from build123d import *

# Parameters (mm, degrees)
SKETCH_1_W               = 114
SKETCH_1_H               = 15
EXTRUDE_1_DEPTH          = 114
FILLET_3_R               = 15
FILLET_4_R               = 2
SKETCH_2_R               = 24
EXTRUDE_2_DEPTH          = 43
FILLET_5_R               = 12
SKETCH_3_R               = 6.5
CUT_EXTRUDE_4_DEPTH      = 167.856225604
SKETCH_3_4_R             = 11
SKETCH_3_4_R_2           = 6.5
CUT_EXTRUDE_5_DEPTH      = 1.5
PATTERN_CIRCULAR_1_COUNT = 4


with BuildPart() as part:
    # Sketch 1 → Extrude 1 (new body)
    with BuildSketch(Plane.XY):
        with Locations((57, -7.5)):
            Rectangle(SKETCH_1_W, SKETCH_1_H)
    extrude(amount=-EXTRUDE_1_DEPTH)

    # Fillet 3
    fillet_3_edges = [part.edges().sort_by_distance(p)[0] for p in [
        (114, -7.5, -114),
        (0, -7.5, -114),
        (114, -7.5, 0),
        (0, -7.5, 0),
    ]]
    fillet(fillet_3_edges, radius=FILLET_3_R)

    # Fillet 4
    fillet_4_edges = [part.edges().sort_by_distance(p)[0] for p in [
        (0, 0, -57),
        (57, 0, -114),
        (57, 0, 0),
        (114, 0, -57),
        (109.606601718, 0, -4.393398282),
        (109.606601718, 0, -109.606601718),
        (4.393398282, 0, -4.393398282),
        (4.393398282, 0, -109.606601718),
    ]]
    fillet(fillet_4_edges, radius=FILLET_4_R)

    # Sketch 2 → Extrude 2 (add)
    with BuildSketch(Plane(origin=(0, 0, 0), x_dir=(1, 0, 0), z_dir=(0, 1, 0))):
        with Locations(Location((57, 57, 0), (0, 0, 270))):
            Circle(SKETCH_2_R)
        with BuildLine():
            ThreePointArc((47.050125629, 56), (67, 57), (47.050125629, 58))
            Line((47.050125629, 58), (43.8, 58))
            Line((43.8, 58), (43.8, 56))
            Line((43.8, 56), (47.050125629, 56))
        make_face(mode=Mode.SUBTRACT)
    extrude(amount=EXTRUDE_2_DEPTH)

    # Fillet 5
    fillet_5_edges = [part.edges().sort_by_distance(p)[0] for p in [
        (57, 0, -81),
    ]]
    fillet(fillet_5_edges, radius=FILLET_5_R)

    # Sketch 3 → Cut-Extrude 4 (cut, through all)
    with BuildSketch(Plane(origin=(0, 0, 0), x_dir=(1, 0, 0), z_dir=(0, 1, 0))):
        with Locations(Location((99, 99.206255551, 0), (0, 0, 270))):
            Circle(SKETCH_3_R)
    cut_extrude_4 = extrude(amount=-CUT_EXTRUDE_4_DEPTH, mode=Mode.SUBTRACT)

    # Sketch 3_4 → Cut-Extrude 5 (cut)
    with BuildSketch(Plane(origin=(0, 0, 0), x_dir=(1, 0, 0), z_dir=(0, 1, 0))):
        with Locations(Location((99, 99.206255551, 0), (0, 0, 270))):
            Circle(SKETCH_3_4_R)
        with Locations(Location((99, 99.206255551, 0), (0, 0, 270))):
            Circle(SKETCH_3_4_R_2, mode=Mode.SUBTRACT)
    cut_extrude_5 = extrude(amount=-CUT_EXTRUDE_5_DEPTH, mode=Mode.SUBTRACT)

    # Pattern Circular 1: Cut-Extrude 4, Cut-Extrude 5 ×4 about axis
    pattern_circular_1_axis = Axis((57, 0, -57), (0, 1, 0))
    add([cut_extrude_4.rotate(pattern_circular_1_axis, i * 360 / PATTERN_CIRCULAR_1_COUNT) for i in range(1, PATTERN_CIRCULAR_1_COUNT)], mode=Mode.SUBTRACT)
    add([cut_extrude_5.rotate(pattern_circular_1_axis, i * 360 / PATTERN_CIRCULAR_1_COUNT) for i in range(1, PATTERN_CIRCULAR_1_COUNT)], mode=Mode.SUBTRACT)


solid = part.part
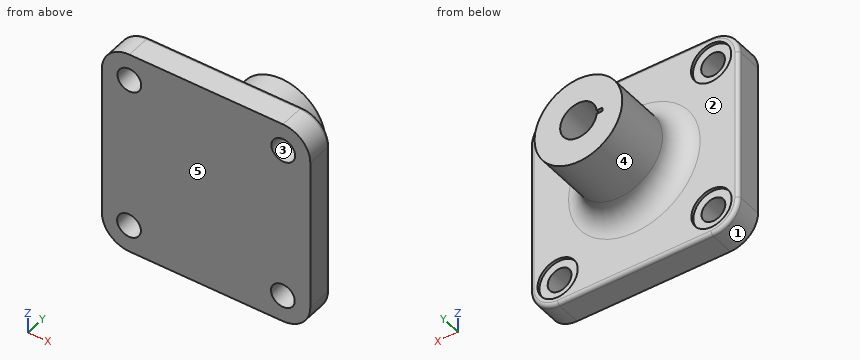
Work out the finished part from the listing and answer in its coordinate system (mm). Face numbers are marked on the shaded views. A direction names the side the tool comes from. Give positions to 0.01 mm unless a question says otherwise; leave off trailing zeros. Loops run counter-clockwise (first coordinate to the right, second up) from the corner with the lowest first, then second, coordinate; pieces in that order, holes last. Notation, with made-up numbers: (-5.5, 45) - (48.5, 45) arc R20 ccw to (48.5, 67) - close; hole circle Ø1 at (72.5, -35). An arc over 180 degrees is marked (long way). Answer in a Markdown table with one row per item.
(1) Section B-B (y = 19.5) is taken. Give the vertices of the cut face in (x, z).
Results list:
| item | result |
|---|---|
| outline | circle Ø48 at (57, -57); hole (43.8, -58) - (47.05, -58) arc R10 ccw (long way) to (47.05, -56) - (43.8, -56) - close |
(2) Section D-D (x = 57) is taken. Give the vertices of the cut face in (y, z).
Results list:
| item | result |
|---|---|
| outline | (-15, -114) - (-2, -114) arc R2 ccw to (0, -112) - (0, -93) arc R12 cw to (12, -81) - (43, -81) - (43, -67) - (0, -67) - (0, -47) - (43, -47) - (43, -33) - (12, -33) arc R12 cw to (0, -21) - (0, -2) arc R2 ccw to (-2, 0) - (-15, 0) - close |
(3) Consider L1, parallel to X at y = -10, z = -99; L2, parallel to Z at x = 15, y = -0.3; L3, parallel to X at y = 12.5, z = -54. Determine where each line is inside the solid, lowest interval first. Write a range as [from, to].
Results list:
| item | result |
|---|---|
| L1 | x = [0, 8.29], [21.29, 92.5], [105.5, 114] |
| L2 | z = [-113.05, -110], [-88, -25.79], [-3.79, -0.95] |
| L3 | x = [33.19, 47.46], [66.54, 80.81] |
(4) A tool of negligible diameter and unlimited length cuts with its end or side. For the marked faces 4 and 5, from which of +Z, -Z, +X, -X, +Y, -Y can it reach the whole face along a straight path? Write none if from no direction.
Results list:
| item | result |
|---|---|
| face 4 | +Y |
| face 5 | +Z, -Z, +X, -X, -Y |
(5) Flat-ended cylindrical pins translate along their axes: pin 1 Ø12 at (x, y) = (15, 1) entering from -Z; pin 2 Ø12 at (y, z) = (37, -91) entering from +X; pin 3 Ø1 at (x, y) = (75, 0) entering from -Z; pin 4 Ø1 at (x, y) = (46, 26) entering from +Z. Find the tip coordinate at first contact, or state that the pin passes through.
Results list:
| item | result |
|---|---|
| pin 1 | stops at z = -114 |
| pin 2 | passes through |
| pin 3 | stops at z = -113.32 |
| pin 4 | stops at z = -35.42 |
(6) Section C-C (x = 96) is taken. Give the vertices of the cut face in (y, z).
Results list:
| item | result |
|---|---|
| outline | (-15, -114) - (-2, -114) arc R2 ccw to (0, -112) - (0, -109.79) - (-1.5, -109.79) - (-1.5, -104.97) - (-15, -104.97) - close; (-15, -93.44) - (-1.5, -93.44) - (-1.5, -88.62) - (0, -88.62) - (0, -25.52) - (-1.5, -25.52) - (-1.5, -20.65) - (-15, -20.65) - close; (-15, -9.35) - (-1.5, -9.35) - (-1.5, -4.48) - (0, -4.48) - (0, -2) arc R2 ccw to (-2, 0) - (-15, 0) - close |
(7) For a pull along X with two mould halves and no side action, classify the marked faces 1, 2 and 3 as pulls with the +X half, pulls with the -X half, needs draft (parallel to the pull), parting line crosses it, or undercut.
Results list:
| item | result |
|---|---|
| face 1 | pulls with the -X half |
| face 2 | needs draft |
| face 3 | undercut |
(8) Section A-A (z = -96.5) is taken. Give the vertices of the cut face in (x, y), and give its area (3 significant figures).
Results list:
| item | result |
|---|---|
| outline | (0, -15) - (8.79, -15) - (8.79, -1.5) - (4.08, -1.5) - (4.08, 0) - (2, 0) arc R2 ccw to (0, -2) - close; (20.79, -15) - (93.09, -15) - (93.09, -1.5) - (88.34, -1.5) - (88.34, 0) - (25.51, 0) - (25.51, -1.5) - (20.79, -1.5) - close; (104.91, -15) - (114, -15) - (114, -2) arc R2 ccw to (112, 0) - (109.66, 0) - (109.66, -1.5) - (104.91, -1.5) - close |
| area | 1,320 mm² |
